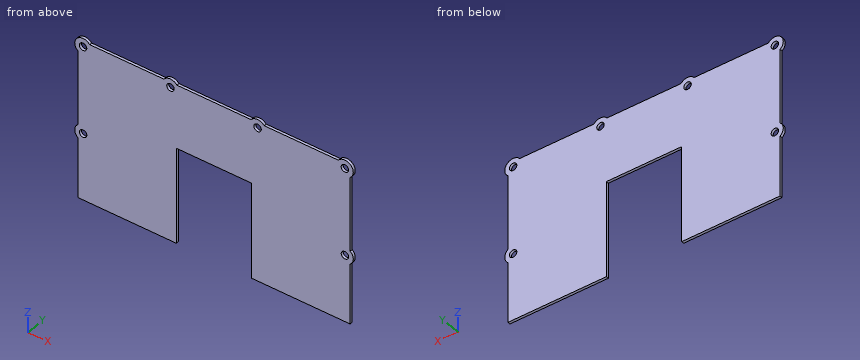
```python
from build123d import *

# Parameters (mm, degrees)
SKETCH1_R           = 2.2479
BOSS_EXTRUDE1_DEPTH = 1.5875


with BuildPart() as part:
    # Sketch1 → Boss-Extrude1 (new body)
    with BuildSketch(Plane(origin=(0, 0, 0), x_dir=(1, 0, 0), z_dir=(0, 1, 0))):
        with BuildLine():
            Line((59.6265, 0), (0, 0))
            Line((0, 0), (0, -36.474509804))
            ThreePointArc((0, -36.474509804), (-1.905, -40.440083533), (0, -44.405657262))
            Line((0, -44.405657262), (0, -89.391176471))
            ThreePointArc((0, -89.391176471), (-0.417102448, -96.948852648), (7.140573729, -96.5317502))
            Line((7.140573729, -96.5317502), (52.126092938, -96.5317502))
            ThreePointArc((52.126092938, -96.5317502), (56.091666667, -98.4367502), (60.057240396, -96.5317502))
            Line((60.057240396, -96.5317502), (63.5, -96.5317502))
            Line((63.5, -96.5317502), (69.85, -96.5317502))
            Line((69.85, -96.5317502), (95.25, -96.5317502))
            Line((95.25, -96.5317502), (101.6, -96.5317502))
            Line((101.6, -96.5317502), (104.917251774, -96.5317502))
            ThreePointArc((104.917251774, -96.5317502), (108.882825503, -98.4367502), (112.848399232, -96.5317502))
            Line((112.848399232, -96.5317502), (157.833918441, -96.5317502))
            ThreePointArc((157.833918441, -96.5317502), (165.391594618, -96.948852648), (164.97449217, -89.391176471))
            Line((164.97449217, -89.391176471), (164.97449217, -44.405657262))
            ThreePointArc((164.97449217, -44.405657262), (166.87949217, -40.440083533), (164.97449217, -36.474509804))
            Line((164.97449217, -36.474509804), (164.97449217, 0))
            Line((164.97449217, 0), (105.34799217, 0))
            Line((105.34799217, 0), (105.34799217, -57.9237502))
            Line((105.34799217, -57.9237502), (59.6265, -57.9237502))
            Line((59.6265, -57.9237502), (59.6265, 0))
        make_face()
        with Locations((3.175, -40.440083533)):
            Circle(SKETCH1_R, mode=Mode.SUBTRACT)
        with Locations((3.175, -93.3567502)):
            Circle(SKETCH1_R, mode=Mode.SUBTRACT)
        with Locations((56.091666667, -93.3567502)):
            Circle(SKETCH1_R, mode=Mode.SUBTRACT)
        with Locations((108.882825503, -93.3567502)):
            Circle(SKETCH1_R, mode=Mode.SUBTRACT)
        with Locations((161.79949217, -93.3567502)):
            Circle(SKETCH1_R, mode=Mode.SUBTRACT)
        with Locations((161.79949217, -40.440083533)):
            Circle(SKETCH1_R, mode=Mode.SUBTRACT)
    extrude(amount=BOSS_EXTRUDE1_DEPTH)


solid = part.part
```
The listing builds one solid part. Answer for the finished solid, in the listing's coordinates (mm). Coordinates: 2 decimals unless noted, no trailing zeros. Loops run counter-clockwise (first coordinate to the right, second up) from the corner with the lowest first, then second, coordinate; pieces in that order, holes last. Notation, with made-up numbers: M -1,34 L 36,34 A19 cw 36,54 Z; hole C 80,58 d2. An arc over 180 degrees is marked long. Answer as CSV lines item,"result". Start each with the question number.
(1) The part is cut by section A-A (z = 18.5). Give the vertices of the cut face in (x, y).
(2) The part is cut by section C-C (x = 93.5). Give the vertices of the cut face in (y, z).
(3) Find the intervals of material crossed by L1, parallel to Z at x = 109, y = 1.45; L2, parallel to X at y = 1.35, z = 16.5; L3, parallel to X at y = 0.7, z = 93.5 (1 decimal), in increasing order. Write a range as [from, to].
(4) The part is cut by section D-D (z = 74). Give the vertices of the cut face in (x, y), and give its area (3 significant figures).
(5) Given pin 1 (4 mm diameter, centred on x = 56.09, z = 93.36, fed in from +Y); pin 2 (0.8 mm diameter, centred on y = 0.5, z = 33, fed in from +X); pin 3 (0.8 mm diameter, centred on x = 134, y = 1, fed in from +Z); pin 4 (0.5 mm diameter, centred on x = 79.5, y = 0.5, fed in from -Z), each flat-ended and moving along its own axis, determine where each tip first touches the part or whether it passes through.
(6) The part is cut by section B-B (y = 1.2). Give the vertices of the cut face in (x, z) (1 decimal), and give its area (3 significant figures).
Determined:
1,outline,"M 0,0 L 59.63,0 L 59.63,1.59 L 0,1.59 Z; M 105.35,0 L 164.97,0 L 164.97,1.59 L 105.35,1.59 Z"
2,outline,"M 0,57.92 L 1.59,57.92 L 1.59,96.53 L 0,96.53 Z"
3,L1,"[0, 91.11], [95.6, 98.44]"
3,L2,"[0, 59.63], [105.35, 164.97]"
3,L3,"[-1.9, 0.9], [5.4, 53.8], [58.3, 106.6], [111.1, 159.6], [164, 166.9]"
4,outline,"M 0,0 L 164.97,0 L 164.97,1.59 L 0,1.59 Z"
4,area,"262 mm2"
5,pin 1,"through"
5,pin 2,"x = 164.97"
5,pin 3,"z = 96.53"
5,pin 4,"z = 57.92"
6,outline,"M 0,0 L 59.6,0 L 59.6,57.9 L 105.3,57.9 L 105.3,0 L 165,0 L 165,36.5 A5.1 ccw 165,44.4 L 165,89.4 A5.1 ccw long 157.8,96.5 L 112.8,96.5 A5.1 ccw 104.9,96.5 L 60.1,96.5 A5.1 ccw 52.1,96.5 L 7.1,96.5 A5.1 ccw long 0,89.4 L 0,44.4 A5.1 ccw 0,36.5 Z; hole C 3.2,40.4 d4.5; hole C 3.2,93.4 d4.5; hole C 56.1,93.4 d4.5; hole C 108.9,93.4 d4.5; hole C 161.8,40.4 d4.5; hole C 161.8,93.4 d4.5"
6,area,"13,300 mm2"
